```python
from build123d import *

# Parameters (mm, degrees)
F1_DEPTH = 19.05
F0_W     = 8.89
F0_H     = 17.78
F2_DEPTH = 3.175


with BuildPart() as f1:
    # F0 (on Top) → F1 (new body)
    with BuildSketch(Plane.XY):
        Polygon((23.5731723178, -23.5731723178), (33.3375, -13.8088446356), (33.3375, 13.8088446356), (23.5731723178, 23.5731723178), (4.445, 8.89), (4.445, -8.89), align=None)
    extrude(amount=F1_DEPTH)



with BuildPart() as f1b:
    # F0 (on Top) → F1, piece 2 (new body)
    with BuildSketch(Plane.XY):
        Polygon((-23.5731723178, -23.5731723178), (-4.445, -8.89), (-4.445, 8.89), (-23.5731723178, 23.5731723178), (-33.3375, 13.8088446356), (-33.3375, -13.8088446356), align=None)
    extrude(amount=F1_DEPTH)


with BuildPart() as f1_1:
    add(f1.part)

    add(f1b.part)  # F2 merges F1b
    # F0 (on Top) → F2 (join)
    with BuildSketch(Plane.XY):
        Rectangle(F0_W, F0_H)
    extrude(amount=F2_DEPTH)


solid = f1_1.part
```
Could you check a few things on this model? Use its own coordinates, in mm. A direction names the side the tool comes from. Coordinates: 2 decimals unless noted, no trailing zeros. Order: outer loops, then holes, each group sorted by start corner. A loop starts at its lowest first (then second) coordinate and runs counter-clockwise, first axis right, second up. Notation, with made-up numbers: M -20.75,42 L 32.25,42 A26 cw 32.25,75 Z; hole C 61,0 d10. An arc over 180 degrees is marked long. Use a Markdown table: item, result. Add a question column.
Q1. If I drill on L1, parallel to X at y = 6, z = 16.75 (1 decimal); L2, parallel to Z at x = 4, y = -7 (3 decimals); L3, parallel to X at y = -11.5, z = 2, over which ranges is the centre line in solid material (lowest first)?
Q2. I want a section at A-A on z = 12.5. List the corners of the cut face in (x, y) for me (1 decimal), then the cut area to 3 significant figures.
Q3. Which directions (+Z, -Z, +X, -X, +Y, -Y) give clear straight access to the entire face, cutting with the end or side of a thin tool? Please do faces 4 (the flat face through (13.88, -16.13, 9.39)), 5 (the flat face through (-4.445, 0, 11)), 6 (the flat face through (-13.88, 16.13, 9.39)).
Q4. I'm going to push flat-ended pins straight in: pin 1 (2.5 mm diameter, centred on x = 0, y = 4, fed in from +Z) (3 decimals); pin 2 (1 mm diameter, centred on x = 21, z = 15, fed in from -Y); pin 3 (1 mm diameter, centred on x = 1, z = 1, fed in from -Y). Where does each tip first touch, or does it pass through?
Q5. I want a section at D-D on x = -14.5. List the corners of the cut face in (y, z) for me.
Q6. We'd pull the mould along X, two halves only. Please class faces 1 (the flat face through (0, 0, 3.175)), 2 (the flat face through (-33.338, 0, 9)), 3 (the flat face through (28.387, -18.759, 9.392)): pulls with the +X half, pulls with the -X half, needs draft (parallel to the pull), parting line crosses it, or undercut.
Q7. I want a section at B-B on y = 12. List the corners of the cut face in (x, z) for me.
Checked values:
| question | item | result |
|---|---|---|
| 1 | L1 | -33.3 to -4.4, 4.4 to 33.3 |
| 1 | L2 | 0 to 3.175 |
| 1 | L3 | -33.34 to -7.85, 7.85 to 33.34 |
| 2 | outline | M -33.3,-13.8 L -23.6,-23.6 L -4.4,-8.9 L -4.4,8.9 L -23.6,23.6 L -33.3,13.8 Z; M 4.4,-8.9 L 23.6,-23.6 L 33.3,-13.8 L 33.3,13.8 L 23.6,23.6 L 4.4,8.9 Z |
| 2 | area | 1,970 mm² |
| 3 | face 4 | +Z, -Z, -Y |
| 3 | face 5 | +Z, +Y, -Y |
| 3 | face 6 | +Z, -Z, +Y |
| 4 | pin 1 | z = 3.175 |
| 4 | pin 2 | y = -21.98 |
| 4 | pin 3 | y = -8.89 |
| 5 | outline | M -16.61,0 L 16.61,0 L 16.61,19.05 L -16.61,19.05 Z |
| 6 | face 1 | undercut |
| 6 | face 2 | pulls with the -X half |
| 6 | face 3 | pulls with the +X half |
| 7 | outline | M -33.34,0 L -8.5,0 L -8.5,19.05 L -33.34,19.05 Z; M 8.5,0 L 33.34,0 L 33.34,19.05 L 8.5,19.05 Z |
